Read the model definition and answer for the solid it produces. Units are mm, in the model's axes. Give positions to 0.01 mm unless a question says otherwise; leave off trailing zeros. Order: outer loops, then holes, each group sorted by start corner. A loop starts at its lowest first (then second) coordinate and runs counter-clockwise, first axis right, second up. Notation, with made-up numbers: (82.5, 41.25) -> (103.5, 41.25) arc R9 ccw to (103.5, 56.25) -> close; hole circle Ø1 at (86.25, 60.5). An arc over 180 degrees is marked (long way). Answer as CSV lines item,"result". Start each with the question number.
1) Find section B-B (z = 16). Determine the outline of the cut face in (x, y).
2) The mould has two halves that part along Z. Classify faces 1 (the face through (-30, -4, 0)), 2 (the face through (29.1, -4.06, 20.14)), 3 (the face through (6, -4, 18)): +Z half, -Z half, draft (parallel to the pull), parting line (faces both ways), or undercut.
3) Straight lines are drawn through the part: L1, parallel to X at y = -2.5, z = -16; L2, parallel to Z at x = 6, y = -5.25; L3, parallel to X at y = -1.5, z = -17. For each, find the intervals that lie inside material, in ascending order. Write a range as from..to.
4) Find section A-A (x = 6). Determine the outline of the cut face in (y, z).
```python
from build123d import *

# Parameters (mm, degrees)
F0_W      = 5
F0_H      = 2.8
F1_DEPTH  = 6.3
F2_W      = 46
F2_H      = 23
F3_DEPTH  = 16
F5_W      = 4
F5_H      = 7.5
F6_DEPTH  = 25
F9_R      = 1.5
F10_W     = 46
F10_H     = 42
F11_DEPTH = 3
F13_R     = 3
F14_W     = 60
F14_H     = 42
F15_DEPTH = 8
F16_R     = 3


with BuildPart() as f1:
    # F0 (on Front) → F1 (new body, symmetric)
    with BuildSketch(Plane.XZ):
        with Locations((14, 6.1)):
            Rectangle(F0_W, F0_H)
        with Locations((-14, 6.1)):
            Rectangle(F0_W, F0_H)
        Polygon((-11.5, -11.5), (11.5, -11.5), (11.5, 4.7), (11.5, 7.5), (11.5, 11.5), (-11.5, 11.5), (-11.5, 7.5), (-11.5, 4.7), align=None)
    extrude(amount=F1_DEPTH, both=True)


with BuildPart() as f3:
    # F2 (on Front) → F3 (new body)
    with BuildSketch(Plane.XZ):
        Rectangle(F2_W, F2_H)
    extrude(amount=F3_DEPTH)


with BuildPart() as f3_1:
    # F4: moved
    add(f3.part.moved(Location((0, 9.75, 0))))


with BuildPart() as f6:
    # F5 (on Front) → F6 (new body)
    with BuildSketch(Plane.XZ):
        with Locations((13.5, -7.75)):
            Rectangle(F5_W, F5_H)
    extrude(amount=F6_DEPTH)


with BuildPart() as f6_1:
    # F7: moved
    add(f6.part.moved(Location((0, 4, 0))))


with BuildPart() as f3_2:
    add(f3_1.part)

    # F8: cut F6, F1
    add(f6_1.part, mode=Mode.SUBTRACT)
    add(f1.part, mode=Mode.SUBTRACT)

    # F9
    f9_edges = [f3_2.edges().sort_by_distance(p)[0] for p in [
        (-23, -6.25, 0),
        (23, -6.25, 0),
        (23, 1.75, 11.5),
        (-23, 1.75, 11.5),
        (-17.25, -6.25, 11.5),
        (17.25, -6.25, 11.5),
        (23, 1.75, -11.5),
        (19.25, -6.25, -11.5),
        (-23, 1.75, -11.5),
        (-17.25, -6.25, -11.5),
    ]]
    fillet(f9_edges, radius=F9_R)


with BuildPart() as f11:
    # F10 (on Front) → F11 (new body)
    with BuildSketch(Plane.XZ):
        Rectangle(F10_W, F10_H)
        with BuildLine():
            Line((-18, -14), (0, -14))
            Line((0, -14), (18, -14))
            ThreePointArc((18, -14), (20, -16), (18, -18))
            Line((18, -18), (-18, -18))
            ThreePointArc((-18, -18), (-20, -16), (-18, -14))
        make_face(mode=Mode.SUBTRACT)
        with BuildLine():
            Line((18, 14), (0, 14))
            Line((0, 14), (-18, 14))
            ThreePointArc((-18, 14), (-20, 16), (-18, 18))
            Line((-18, 18), (18, 18))
            ThreePointArc((18, 18), (20, 16), (18, 14))
        make_face(mode=Mode.SUBTRACT)
    extrude(amount=F11_DEPTH)


with BuildPart() as f11_1:
    # F12: moved
    add(f11.part.moved(Location((0, 12, 0))))

    # F13
    f13_edges = [f11_1.edges().sort_by_distance(p)[0] for p in [
        (-23, 10.5, 21),
        (23, 10.5, 21),
        (23, 10.5, -21),
        (-23, 10.5, -21),
    ]]
    fillet(f13_edges, radius=F13_R)


with BuildPart() as f15:
    # F14 (on Front) → F15 (new body)
    with BuildSketch(Plane.XZ):
        Rectangle(F14_W, F14_H)
        with BuildLine():
            ThreePointArc((2, -16), (-1.4142135624, -17.4142135624), (0, -14))
            ThreePointArc((0, -14), (1.4142135624, -14.5857864376), (2, -16))
        make_face(mode=Mode.SUBTRACT)
        with BuildLine():
            ThreePointArc((8, 16), (6, 14), (4, 16))
            ThreePointArc((4, 16), (6, 18), (8, 16))
        make_face(mode=Mode.SUBTRACT)
    extrude(amount=F15_DEPTH)

    # F16
    f16_edges = [f15.edges().sort_by_distance(p)[0] for p in [
        (30, -4, -21),
        (-30, -4, -21),
        (-30, -4, 21),
        (30, -4, 21),
    ]]
    fillet(f16_edges, radius=F16_R)


solid = f15.part
```
Findings below:
1,outline,"(-30, -8) -> (4, -8) -> (4, 0) -> (-30, 0) -> close; (8, -8) -> (30, -8) -> (30, 0) -> (8, 0) -> close"
2,face 1,"draft"
2,face 2,"+Z half"
2,face 3,"undercut"
3,L1,"-30..-2, 2..30"
3,L2,"-21..14, 18..21"
3,L3,"-30..-1.73, 1.73..30"
4,outline,"(-8, -21) -> (0, -21) -> (0, 14) -> (-8, 14) -> close; (-8, 18) -> (0, 18) -> (0, 21) -> (-8, 21) -> close"
